CAD build for the part. Positions are in the model's coordinates, mm. A direction names the side the tool comes from. Give positions to 0.01 mm unless a question says otherwise; leave off trailing zeros. Loops run counter-clockwise (first coordinate to the right, second up) from the corner with the lowest first, then second, coordinate; pieces in that order, holes last. Notation, with made-up numbers: (-37, 69) -> (20, 69) arc R16 ccw to (20, 94) -> close; hole circle Ø11 at (-30, 37.5). An arc over 180 degrees is marked (long way). Write each question's results on one line, items separated by ' | '. Start each with the question number.
```python
from build123d import *

# Parameters (mm, degrees)
SKETCH1_R            = 1.45
BOSS_EXTRUDE1_DEPTH  = 8.5
BOSS_EXTRUDE2_START  = -8.5
BOSS_EXTRUDE2_DEPTH  = 8.5
BOSS_EXTRUDE3_DEPTH  = 10
SKETCH4_R            = 5
BOSS_EXTRUDE4_DEPTH  = 10
BOSS_EXTRUDE5_DEPTH  = 10
BOSS_EXTRUDE6_DEPTH  = 10
BOSS_EXTRUDE7_DEPTH  = 10
BOSS_EXTRUDE8_DEPTH  = 10
BOSS_EXTRUDE9_DEPTH  = 10
SKETCH10_R           = 1.45
CUT_EXTRUDE2_DEPTH   = 28
SKETCH11_W           = 6.5
SKETCH11_H           = 22.932404029
SKETCH11_H_2         = 5
SKETCH11_H_3         = 8.694974759
CUT_EXTRUDE3_DEPTH   = 49
SKETCH12_W           = 6.5
SKETCH12_H           = 22.932404029
CUT_EXTRUDE4_DEPTH   = 49
SKETCH14_W           = 6.5
SKETCH14_H           = 20.273775142
CUT_EXTRUDE5_DEPTH   = 49
BOSS_EXTRUDE10_START = 1.25
SKETCH17_R           = 2.5
SKETCH17_R_2         = 1.45
BOSS_EXTRUDE10_DEPTH = 1.25
SKETCH18_R           = 2.5
SKETCH18_R_2         = 1.45
BOSS_EXTRUDE11_DEPTH = 1.25
SKETCH19_R           = 2.5
BOSS_EXTRUDE12_DEPTH = 1.25
BOSS_EXTRUDE13_START = 1.25
SKETCH21_R           = 2.5
SKETCH21_R_2         = 1.45
BOSS_EXTRUDE13_DEPTH = 1.25
SKETCH22_R           = 1.45
CUT_EXTRUDE6_DEPTH   = 70.556228756


with BuildPart() as part:
    # Sketch1 → Boss-Extrude1 (new body)
    with BuildSketch(Plane(origin=(0, 0, 0), x_dir=(0, 0, -1), z_dir=(1, 0, 0))):
        with BuildLine():
            Line((27, 10), (5, 10))
            ThreePointArc((5, 10), (0, 5), (5, 0))
            Line((5, 0), (27, 0))
            ThreePointArc((27, 0), (32, 5), (27, 10))
        make_face()
        with Locations((5, 5)):
            Circle(SKETCH1_R, mode=Mode.SUBTRACT)
        with Locations((27, 5)):
            Circle(SKETCH1_R, mode=Mode.SUBTRACT)
    extrude(amount=BOSS_EXTRUDE1_DEPTH)

    # Sketch2 → Boss-Extrude2 (add)
    with BuildSketch(Plane(origin=(8.5, 0, 0), x_dir=(0, 0, -1), z_dir=(1, 0, 0)).offset(BOSS_EXTRUDE2_START)):
        with BuildLine():
            add(Edge.make_bspline(
                [(63.752972286, 17.872423117), (45.928882678, 26.563787963), (31.059268621, 10), (13.694974759, 10)],
                knots=[0, 0, 0, 0, 1, 1, 1, 1], degree=3))
            Line((13.694974759, 10), (27, 10))
            ThreePointArc((27, 10), (31.87285141, 6.120410255), (29.183837075, 0.502127655))
            Line((29.183837075, 0.502127655), (38.08542066, 4.824084077))
            add(Edge.make_bspline(
                [(38.08542066, 4.824084077), (46.797509509, 11.895222457), (57.948000409, 11.067843667)],
                knots=[0, 0, 0, 1, 1, 1], degree=2))
            Line((57.948000409, 11.067843667), (65.313809691, 14.189518476))
            Line((65.313809691, 14.189518476), (63.752972286, 17.872423117))
        make_face()
    extrude(amount=BOSS_EXTRUDE2_DEPTH)

    # Sketch3 → Boss-Extrude3 (add)
    with BuildSketch(Plane(origin=(8.5, 0, 0), x_dir=(0, 0, -1), z_dir=(1, 0, 0))):
        with BuildLine():
            Line((36.108074214, 3.8640296), (33.121739514, 15.047376099))
            add(Edge.make_bspline(
                [(63.752972286, 17.872423117), (52.853080786, 23.187417369), (43.058056373, 19.057897142), (33.121739514, 15.047376099)],
                knots=[0, 0, 0, 0, 0.611525847, 0.611525847, 0.611525847, 0.611525847], degree=3))
            Line((63.752972286, 17.872423117), (65.313809691, 14.189518476))
            Line((65.313809691, 14.189518476), (57.948000409, 11.067843667))
            add(Edge.make_bspline(
                [(38.08542066, 4.824084077), (46.79750951, 11.895222457), (57.948000409, 11.067843667)],
                knots=[0, 0, 0, 1, 1, 1], degree=2))
            Line((38.08542066, 4.824084077), (36.108074214, 3.8640296))
        make_face()
    extrude(amount=BOSS_EXTRUDE3_DEPTH)

    # Sketch4 → Boss-Extrude4 (add)
    with BuildSketch(Plane(origin=(8.5, 0, 0), x_dir=(0, 0, -1), z_dir=(1, 0, 0))):
        with Locations(Location((5, 5, 0), (0, 0, 270))):
            Circle(SKETCH4_R)
    extrude(amount=BOSS_EXTRUDE4_DEPTH)

    # Sketch5 → Boss-Extrude5 (add)
    with BuildSketch(Plane(origin=(8.5, 0, 0), x_dir=(0, 0, -1), z_dir=(1, 0, 0))):
        with BuildLine():
            Line((5, 10), (13.694974759, 10))
            Line((13.694974759, 10), (13.694974759, 0))
            Line((13.694974759, 0), (5, 0))
            ThreePointArc((5, 0), (10, 5), (5, 10))
        make_face()
    extrude(amount=BOSS_EXTRUDE5_DEPTH)

    # Sketch6 → Boss-Extrude6 (add)
    with BuildSketch(Plane(origin=(8.5, 0, 0), x_dir=(0, 0, -1), z_dir=(1, 0, 0))):
        with BuildLine():
            Line((19.355254229, 10.548091727), (21.320062705, 0))
            Line((21.320062705, 0), (13.694974759, 0))
            Line((13.694974759, 0), (13.694974759, 10))
            add(Edge.make_bspline(
                [(19.355254229, 10.548091727), (17.493954956, 10.201384788), (15.609630186, 10), (13.694974759, 10)],
                knots=[0.889736062, 0.889736062, 0.889736062, 0.889736062, 1, 1, 1, 1], degree=3))
        make_face()
    extrude(amount=BOSS_EXTRUDE6_DEPTH)

    # Sketch7 → Boss-Extrude7 (add)
    with BuildSketch(Plane(origin=(8.5, 0, 0), x_dir=(0, 0, -1), z_dir=(1, 0, 0))):
        with BuildLine():
            Line((32.645955645, 2.183078628), (28.509427835, 13.235241807))
            add(Edge.make_bspline(
                [(33.121739514, 15.047376099), (31.589187648, 14.428803684), (30.053274551, 13.813062163), (28.509427835, 13.235241807)],
                knots=[0.611525847, 0.611525847, 0.611525847, 0.611525847, 0.705846016, 0.705846016, 0.705846016, 0.705846016], degree=3))
            Line((33.121739514, 15.047376099), (36.108074214, 3.8640296))
            Line((36.108074214, 3.8640296), (32.645955645, 2.183078628))
        make_face()
    extrude(amount=BOSS_EXTRUDE7_DEPTH)

    # Sketch8 → Boss-Extrude8 (add)
    with BuildSketch(Plane(origin=(8.5, 0, 0), x_dir=(0, 0, -1), z_dir=(1, 0, 0))):
        with BuildLine():
            Line((27, 0), (23.604335966, 11.578089924))
            add(Edge.make_bspline(
                [(28.509427835, 13.235241807), (26.884956708, 12.627245898), (25.251701682, 12.061235292), (23.604335966, 11.578089924)],
                knots=[0.705846016, 0.705846016, 0.705846016, 0.705846016, 0.805091873, 0.805091873, 0.805091873, 0.805091873], degree=3))
            Line((28.509427835, 13.235241807), (32.645955645, 2.183078628))
            Line((32.645955645, 2.183078628), (29.183837075, 0.502127655))
            ThreePointArc((29.183837075, 0.502127655), (28.120410255, 0.12714859), (27, 0))
        make_face()
    extrude(amount=BOSS_EXTRUDE8_DEPTH)

    # Sketch9 → Boss-Extrude9 (add)
    with BuildSketch(Plane(origin=(8.5, 0, 0), x_dir=(0, 0, -1), z_dir=(1, 0, 0))):
        with BuildLine():
            Line((23.604335966, 11.578089924), (27, 0))
            Line((27, 0), (21.320062705, 0))
            Line((21.320062705, 0), (19.355254229, 10.548091727))
            add(Edge.make_bspline(
                [(19.355254229, 10.548091727), (20.788925962, 10.815127802), (22.205425846, 11.167809658), (23.604335966, 11.578089924)],
                knots=[0, 0, 0, 0, 1, 1, 1, 1], degree=3))
        make_face()
    extrude(amount=BOSS_EXTRUDE9_DEPTH)

    # Sketch10 → Cut-Extrude2 (cut)
    with BuildSketch(Plane.ZY):
        with Locations(Location((-27, 5, 0), (0, 0, 180))):
            Circle(SKETCH10_R)
        with Locations(Location((-5, 5, 0), (0, 0, 180))):
            Circle(SKETCH10_R)
    extrude(amount=-CUT_EXTRUDE2_DEPTH, mode=Mode.SUBTRACT)

    # Sketch11 → Cut-Extrude3 (cut)
    with BuildSketch(Plane(origin=(0, 10, 0), x_dir=(1, 0, 0), z_dir=(0, 1, 0))):
        with Locations((9.25, 25.161176774)):
            Rectangle(SKETCH11_W, SKETCH11_H)
        with Locations((9.25, 2.5)):
            Rectangle(SKETCH11_W, SKETCH11_H_2)
        with Locations((9.25, 9.34748738)):
            Rectangle(SKETCH11_W, SKETCH11_H_3)
    extrude(amount=-CUT_EXTRUDE3_DEPTH, mode=Mode.SUBTRACT)

    # Sketch12 → Cut-Extrude4 (cut)
    with BuildSketch(Plane(origin=(0, 10, 0), x_dir=(-1, 0, 0), z_dir=(0, -1, 0))):
        with Locations((-9.25, 25.161176774)):
            Rectangle(SKETCH12_W, SKETCH12_H)
    extrude(amount=-CUT_EXTRUDE4_DEPTH, mode=Mode.SUBTRACT)

    # Sketch14 → Cut-Extrude5 (cut)
    with BuildSketch(Plane.XZ):
        with Locations((9.25, -50.780431109)):
            Rectangle(SKETCH14_W, SKETCH14_H)
    extrude(amount=-CUT_EXTRUDE5_DEPTH, mode=Mode.SUBTRACT)

    # Sketch17 → Boss-Extrude10 (add)
    with BuildSketch(Plane.ZY.offset(-12.5).offset(BOSS_EXTRUDE10_START)):
        with Locations(Location((-5, 5, 0), (0, 0, 180))):
            Circle(SKETCH17_R)
        with Locations(Location((-5, 5, 0), (0, 0, 180))):
            Circle(SKETCH17_R_2, mode=Mode.SUBTRACT)
    extrude(amount=-BOSS_EXTRUDE10_DEPTH)

    # Sketch18 → Boss-Extrude11 (add)
    with BuildSketch(Plane(origin=(6, 0, 0), x_dir=(0, 0, -1), z_dir=(1, 0, 0))):
        with Locations((5, 5)):
            Circle(SKETCH18_R)
        with Locations((5, 5)):
            Circle(SKETCH18_R_2, mode=Mode.SUBTRACT)
    extrude(amount=BOSS_EXTRUDE11_DEPTH)

    # Sketch19 → Boss-Extrude12 (add)
    with BuildSketch(Plane(origin=(6, 0, 0), x_dir=(0, 0, -1), z_dir=(1, 0, 0))):
        with Locations((27, 5)):
            Circle(SKETCH19_R)
    extrude(amount=BOSS_EXTRUDE12_DEPTH)

    # Sketch21 → Boss-Extrude13 (add)
    with BuildSketch(Plane.ZY.offset(-12.5).offset(BOSS_EXTRUDE13_START)):
        with Locations(Location((-27, 5, 0), (0, 0, 180))):
            Circle(SKETCH21_R)
        with Locations(Location((-27, 5, 0), (0, 0, 180))):
            Circle(SKETCH21_R_2, mode=Mode.SUBTRACT)
    extrude(amount=-BOSS_EXTRUDE13_DEPTH)

    # Sketch22 → Cut-Extrude6 (cut, through all)
    with BuildSketch(Plane.ZY.offset(-12.5)):
        with Locations(Location((-27, 5, 0), (0, 0, 180))):
            Circle(SKETCH22_R)
    extrude(amount=CUT_EXTRUDE6_DEPTH, mode=Mode.SUBTRACT)


solid = part.part
```
Q1. Wall check: L1, parallel to X at y = 6.5, z = -33.5; L2, parallel to Y at x = 6.9, z = -5; L3, parallel to Z at x = 16.5, y = 5. Give the ranges that are in metal, low to high.
Q2. Drop flat-ended pins along their axis: pin 1 (4 mm diameter, centred on x = 4, y = 2.5, fed in from +Z); pin 2 (4.5 mm diameter, centred on y = 5, z = -5, fed in from +X); pin 3 (1 mm diameter, centred on x = 9, y = 7, fed in from -Z); pin 4 (1.7 mm diameter, centred on y = 5, z = -27, fed in from +X). Give the stop position or say it passes through.
Q3. Saw through at A-A, the plane z = -10. List the corners of the cut face in (x, y), then the cut area to 3 significant figures.
Q4. Which spindle directions (+Z, -Z, +X, -X, +Y, -Y) get a long thin tool onto all of the face, cutting with end or side? Do faces 5 (the face through (11.25, 5, -7)), 6 (the face through (6.62, 6.69, -25.16)), 7 (the face through (9, 12, -40.644)), 8 (the face through (15, 10, -9)). Say none if no direction does.
Q5. Mould opens along Z. For faces 1 (the face through (11.25, 5, -29)), 2 (the face through (12.5, 15, -51)), 3 (the face through (15.46, 0.13, -28.14)), 4 (the face through (3, 5, 0)) say: pulls with the +Z half, pulls with the -Z half, needs draft (parallel to the pull), parting line crosses it, or undercut.
Q6. Saw through at B-B, the plane x = 15.5. Give the number of separate pieces and of enclosed holes in the cut face, then the cut area to 3 significant figures.
Answer block:
1) L1: x = 0 to 6, 12.5 to 18.5 | L2: y = 2.5 to 3.55, 6.45 to 7.5 | L3: z = -38.3 to -28.45, -25.55 to -6.45, -3.55 to 0
2) pin 1: stops at z = -0.03 | pin 2: stops at x = 18.5 | pin 3: stops at z = -40.64 | pin 4: passes through
3) outline: (0, 0) -> (6, 0) -> (6, 10) -> (0, 10) -> close; (12.5, 0) -> (18.5, 0) -> (18.5, 10) -> (12.5, 10) -> close | area: 120 mm2
4) face 5: +Z, +Y, -Y | face 6: none | face 7: +Y, -Y | face 8: +Z, +X, -X, +Y
5) face 1: needs draft | face 2: undercut | face 3: pulls with the -Z half | face 4: pulls with the +Z half
6) separate pieces: 1 | enclosed holes: 2 | area: 641 mm2
